Verification items for this drawing (mm, ordinates from the low corner). A direction names the side the tool comes from. Coordinates: 2 decimals unless noted, no trailing zeros. Write each loop counter-clockwise with the first axis right and the second up, starting at its lowest first coordinate (ties: lowest second). Pieces come first, ordered by that corner, then holes. Notation, with made-up numbers: (50.25, 19) -> (63.25, 19) arc R16 cw to (63.25, 49) -> close; hole circle Ø5 at (61, 25.25). An arc over 180 degrees is marked (long way). Use CSV: the item, a comma, the result in double quotes.
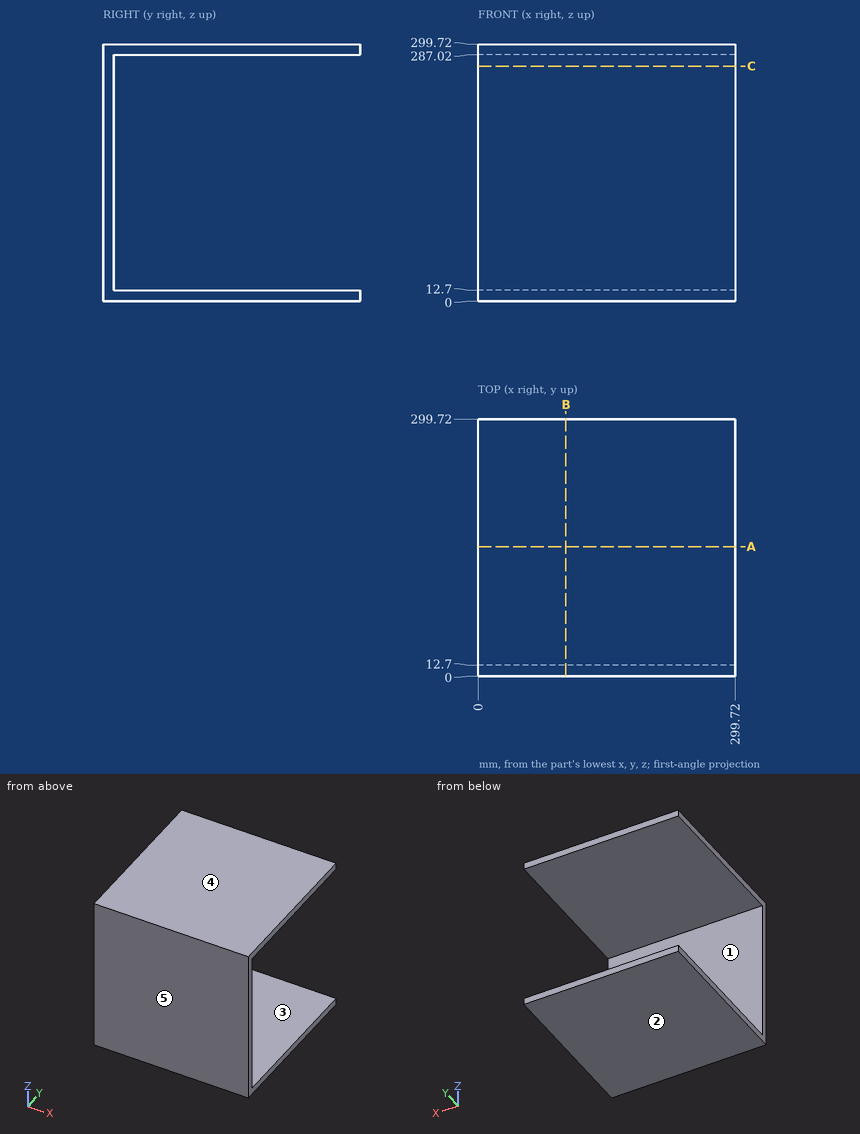
1) Set-up check for the marked faces 1 and 2: record each of +Z, -Z, +X, -X, +Y, -Y from which the full face is reachable in a straight line by a thin tool's end or side.
Return value:
face 1,"+X, -X, +Y"
face 2,"-Z, +X, -X, +Y, -Y"
2) Cross-section at C-C (z = 274). Record the boundary of the cut face in (x, y).
Return value:
outline,"(0, 0) -> (299.72, 0) -> (299.72, 12.7) -> (0, 12.7) -> close"
3) Mould release check, pull along Z, two halves, no side actions. Record for the marked faces 3, 4 and 5: released by +Z, released by -Z, zero draft, split by the parting line, or undercut.
Return value:
face 3,"undercut"
face 4,"released by +Z"
face 5,"zero draft"
4) Cross-section at B-B (x = 102.5). Record the boundary of the cut face in (y, z).
Return value:
outline,"(0, 0) -> (299.72, 0) -> (299.72, 12.7) -> (12.7, 12.7) -> (12.7, 287.02) -> (299.72, 287.02) -> (299.72, 299.72) -> (0, 299.72) -> close"
5) Scan lines: L1, parallel to Z at x = 19, y = 54; L2, parallel to Y at x = 202.5, z = 167. Record each from-to range of solid material in increasing order.
Return value:
L1,"0 to 12.7, 287.02 to 299.72"
L2,"0 to 12.7"
6) Gauge pin test, flat end, axial feed: pin 1 (4 mm diameter, centred on x = 150.5, z = 109, fed in from +Y). Record the tip position at first contact, or that the pin passes through.
Return value:
pin 1,"y = 12.7"
7) Cross-section at A-A (y = 151). Record the boundary of the cut face in (x, z).
Return value:
outline,"(0, 0) -> (299.72, 0) -> (299.72, 12.7) -> (0, 12.7) -> close; (0, 287.02) -> (299.72, 287.02) -> (299.72, 299.72) -> (0, 299.72) -> close"
